Here's how the part is built. I have some questions about the finished solid (model axes, mm). A direction names the side the tool comes from. Give positions to 0.01 mm unless a question says otherwise; leave off trailing zeros. Write each loop counter-clockwise with the first axis right and the second up, starting at its lowest first coordinate (ties: lowest second). Pieces come first, ordered by that corner, then holes. Notation, with made-up numbers: M 72.5,13 L 89.5,13 A15 cw 89.5,21 Z; hole C -33,45 d7. An arc over 180 degrees is marked long. Use one line per item in the form item = value. Start each with the question number.
from build123d import *

# Parameters (mm, degrees)
SKETCH6_W           = 36.322
SKETCH6_H           = 7.14375
EXTRUDE1_DEPTH      = 7.874
SKETCH7_W           = 36.322
SKETCH7_H           = 3.81
SKETCH17_R          = 7.14375
CUT_EXTRUDE1_DEPTH  = 14.224
SKETCH19_R          = 6.858
BOSS_EXTRUDE1_DEPTH = 14.224
BOSS_EXTRUDE1_TAPER = 1.75
CHAMFER1_SIZE2      = 1.058333333
CHAMFER1_SIZE       = 1.092196811
SKETCH22_R          = 6.858
BOSS_EXTRUDE3_DEPTH = 14.224
BOSS_EXTRUDE3_TAPER = 15
SKETCH23_R          = 3.556
CUT_EXTRUDE2_DEPTH  = 14.224


with BuildPart() as part:
    # Sketch6 → Revolve3 (revolve)
    with BuildSketch(Plane.XY):
        with Locations((0, 3.571875)):
            Rectangle(SKETCH6_W, SKETCH6_H)
    revolve(axis=Axis((-18.161, 0, 0), (1, 0, 0)))

    # Sketch12 → Extrude1 (add)
    with BuildSketch(Plane(origin=(-3.937, 0, 0), x_dir=(0, 0, -1), z_dir=(1, 0, 0))):
        Polygon((0, 9.165435523), (-7.9375, 4.582717762), (-7.9375, -4.582717762), (0, -9.165435523), (7.9375, -4.582717762), (7.9375, 4.582717762), align=None)
    extrude(amount=EXTRUDE1_DEPTH)

    # Sketch10 → Cut-Revolve6 (revolve, cut)
    with BuildSketch(Plane.XY):
        Polygon((6.038876886, 7.14375), (3.937, 7.14375), (3.937, 6.100206448), (4.995333333, 6.100206448), align=None)
        Polygon((18.161, 7.14375), (12.214385213, 7.14375), (13.257928765, 6.100206448), (15.374595432, 6.100206448), (18.161, 4.0005), align=None)
    revolve(axis=Axis((-18.161, 0, 0), (1, 0, 0)), mode=Mode.SUBTRACT)

    # Sketch7 → Cut-Revolve5 (revolve, cut)
    with BuildSketch(Plane.XY):
        with Locations((0, 1.905)):
            Rectangle(SKETCH7_W, SKETCH7_H)
    revolve(axis=Axis((18.161, 0, 0), (-1, 0, 0)), mode=Mode.SUBTRACT)

    # Sketch13 → Cut-Revolve7 (revolve, cut)
    with BuildSketch(Plane.XY):
        Polygon((-3.937, 9.165435523), (-3.937, 7.9375), (-3.228051095, 9.165435523), align=None)
        Polygon((3.228051095, 9.165435523), (3.937, 7.9375), (3.937, 9.165435523), align=None)
    revolve(axis=Axis((-18.161, 0, 0), (1, 0, 0)), mode=Mode.SUBTRACT)

    # Sketch17 → Cut-Extrude1 (cut)
    with BuildSketch(Plane.ZY.offset(18.161)):
        Circle(SKETCH17_R)
    extrude(amount=-CUT_EXTRUDE1_DEPTH, mode=Mode.SUBTRACT)


with BuildPart() as body_2:
    # Sketch19 → Boss-Extrude1 (new body)
    with BuildSketch(Plane(origin=(-3.937, 0, 0), x_dir=(0, 0, -1), z_dir=(1, 0, 0))):
        Circle(SKETCH19_R)
    extrude(amount=-BOSS_EXTRUDE1_DEPTH, taper=BOSS_EXTRUDE1_TAPER)

    # Chamfer1
    chamfer1_edges = [body_2.edges().sort_by_distance(p)[0] for p in [
        (-18.161, 0, 6.423417495),
    ]]
    chamfer(chamfer1_edges, length=CHAMFER1_SIZE, length2=CHAMFER1_SIZE2)

    # Sketch22 → Boss-Extrude3 (add)
    with BuildSketch(Plane(origin=(-3.937, 0, 0), x_dir=(0, 0, -1), z_dir=(1, 0, 0))):
        Circle(SKETCH22_R)
    extrude(amount=-BOSS_EXTRUDE3_DEPTH, taper=BOSS_EXTRUDE3_TAPER)

    # Combine1: union part
    add(part.part)

    # Sketch23 → Cut-Extrude2 (cut)
    with BuildSketch(Plane.ZY.offset(18.161)):
        Circle(SKETCH23_R)
    extrude(amount=-CUT_EXTRUDE2_DEPTH, mode=Mode.SUBTRACT)


solid = body_2.part
1) On a 3-axis mill with a long thin cutter (end or side, diameter ignored), from which of +Z, -Z, +X, -X, +Y, -Y can I reach the whole of each face in a straight line? I mean faces 4 (the face through (-18.161, -4, -1)), 5 (the face through (3.937, -6, 2)). Say none if no direction works.
2) Suppose I cut it at C-C, the plane x = -4.5. List the corners of the cut face in (y, z) for me.
3) Suppose I cut it at B-B, the plane x = 8. List the corners of the cut face in (y, z) for me.
4) Thinking about a two-plate mould opening in Z: for faces 1 (the face through (-0.055, -6.842, 4.024)), 2 (the face through (-3.937, -2, 7)), 3 (the face through (-11.15, -3.47, -0.77)), which applies, released by +Z, released by -Z, zero draft, split by the parting line, or undercut?
5) Suppose I cut it at A-A, the plane x = 1. List the corners of the cut face in (y, z) for me, and give its area (3 significant figures).
6) Please list where these lines run through material, in increasing order: line 1 (Z direction, x = 8.5, y = 0); line 2 (Y direction, x = 1.25, z = 0); line 3 (Y direction, x = -6, z = -0.75).
7) Will these pins go through, and if not, where does the flat tip stop? P1, Ø2, axis at x = -11.5, y = -4.5, coming from the +Z side; P2, Ø9, axis at y = 0, z = 0, coming from the +X side; P3, Ø5, axis at x = -10, z = 6, coming from the +Y side; P4, Ø4.5, axis at y = 0, z = 0, coming from the +X side.
Checks:
q1.face_4 = +Z, -Z, -X, +Y, -Y
q1.face_5 = none
q2.outline = C 0,0 d13.68; hole C 0,0 d7.11
q3.outline = C 0,0 d14.29; hole C 0,0 d7.62
q4.face_1 = released by +Z
q4.face_2 = zero draft
q4.face_3 = undercut
q5.outline = M -9.17,0 L -4.58,-7.94 L 4.58,-7.94 L 9.17,0 L 4.58,7.94 L -4.58,7.94 Z; hole C 0,0 d7.62
q5.area = 173 mm^2
q6.line_1 = -7.14 to -3.81, 3.81 to 7.14
q6.line_2 = -9.17 to -3.81, 3.81 to 9.17
q6.line_3 = -6.75 to -3.48, 3.48 to 6.75
q7.P1 = 5.63
q7.P2 = 18.16
q7.P3 = 5.68
q7.P4 = through
